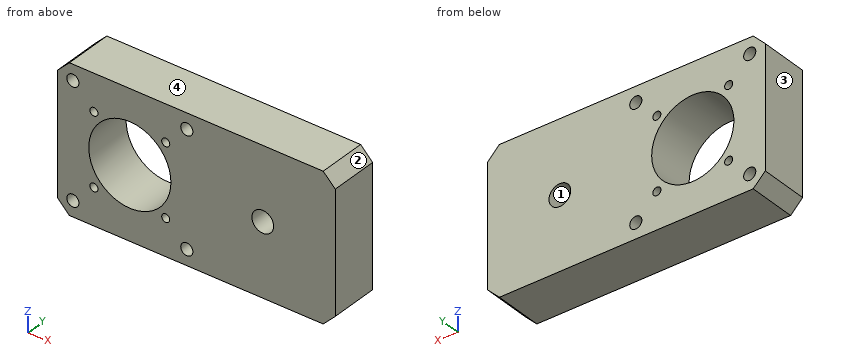
Autodesk Fusion 360 part; units mm, degrees
sketch "Sketch1" plane through (0, 0, 0) normal (0, 1, 0) x (1, 0, 0)
  circle A0 centre (-55, 0) radius 17
  line L0 (-78.57, 23.57) -> (-31.43, 23.57) construction
  line L1 (-31.43, 23.57) -> (-31.43, -23.57) construction
  line L2 (-31.43, -23.57) -> (-78.57, -23.57) construction
  line L3 (-78.57, -23.57) -> (-78.57, 23.57) construction
  line L4 (-78.57, -23.57) -> (-31.43, 23.57) construction
  line L5 (-85, 30) -> (30, 30)
  line L6 (30, 30) -> (30, -30)
  line L7 (30, -30) -> (-85, -30)
  line L8 (-85, -30) -> (-85, 30)
  line L9 (0, 0) -> (-55, 0) construction
  circle A1 centre (-55, 0) radius 21 construction
  line L10 (-78.57, 23.57) -> (-31.43, -23.57) construction
  line L11 (-55, 23.57) -> (-55, -23.57) construction
  line L12 (-78.57, 0) -> (-31.43, 0) construction
  point P0 (-55, 21)
  point P1 (-69.8492, 14.8492)
  point P2 (-76, 0)
  point P3 (-69.8492, -14.8492)
  point P4 (-55, -21)
  point P5 (-40.1508, -14.8492)
  point P6 (-40.1508, 14.8492)
  point P7 (-34, 0)
  dimension "d2" = 34
  dimension "d3" = 55
  dimension "d4" = 47.14
  dimension "d5" = 30
  dimension "d6" = 30
  dimension "d7" = 60
  dimension "d20" = 42
extrude "Extrude1" add sketch "Sketch1" along normal blind 20
hole "Hole1" at (0, 0, 0) direction (0, 1, 0) diameter 9 end through all
hole "Hole2" at (-31.43, 0, 23.57) at (-31.43, 0, -23.57) at (-78.57, 0, -23.57) at (-78.57, 0, 23.57) direction (0, 1, 0) diameter 5.029 end through all
hole "Hole3" at (-69.8492, 0, 14.8492) at (-69.8492, 0, -14.8492) at (-40.1508, 0, -14.8492) at (-40.1508, 0, 14.8492) direction (0, 1, 0) diameter 3.332 end through all
chamfer "Chamfer3" distance 5 angle 45 4 edges at (-85, 10, 30) (-85, 10, -30) (30, 10, 30) (30, 10, -30)
Work out the finished part from the listing and answer in its coordinate system (mm). Face numbers are marked on the shaded views. Give positions to 0.01 mm unless a question says otherwise; leave off trailing zeros. Order: outer loops, then holes, each group sorted by start corner. A loop starts at its lowest first (then second) coordinate and runs counter-clockwise, first axis right, second up.
1. Section A-A, the plane x = -31.43 is taken. Determine the outline of the cut face in (y, z).
Result sheet:
outline: (0, -30) - (20, -30) - (20, -26.08) - (0, -26.08) - close; (0, -21.06) - (20, -21.06) - (20, 21.06) - (0, 21.06) - close; (0, 26.08) - (20, 26.08) - (20, 30) - (0, 30) - close
2. Straight lines are drawn through the part: L1, parallel to X at y = 11.5, z = -23.57; L2, parallel to X at y = 5.25, z = 0; L3, parallel to Z at x = -79, y = 3.75. For each, find the intervals that lie inside material, in ascending order.
Result sheet:
L1: x = -85 to -81.08, -76.06 to -33.94, -28.92 to 30
L2: x = -85 to -72, -38 to -4.5, 4.5 to 30
L3: z = -30 to -26.05, -21.09 to 21.09, 26.05 to 30
3. Section D-D, the plane z = -8 is taken. Determine the outline of the cut face in (x, y).
Result sheet:
outline: (-85, 0) - (-70, 0) - (-70, 20) - (-85, 20) - close; (-40, 0) - (30, 0) - (30, 20) - (-40, 20) - close
4. Section B-B, the plane x = -55 is taken. Determine the outline of the cut face in (y, z).
Result sheet:
outline: (0, -30) - (20, -30) - (20, -17) - (0, -17) - close; (0, 17) - (20, 17) - (20, 30) - (0, 30) - close
5. Section C-C, the plane z = 0 is taken. Determine the outline of the cut face in (x, y).
Result sheet:
outline: (-85, 0) - (-72, 0) - (-72, 20) - (-85, 20) - close; (-38, 0) - (-4.5, 0) - (-4.5, 20) - (-38, 20) - close; (4.5, 0) - (30, 0) - (30, 20) - (4.5, 20) - close
6. The mould has two halves that part along X. Classify the marked faces 1, 2, 3 and 4: released by +X, released by -X, zero draft, split by the parting line, or undercut.
Result sheet:
face 1: undercut
face 2: released by +X
face 3: released by -X
face 4: zero draft
